```python
from build123d import *

# Parameters (mm, degrees)
EXTRUIR1_DEPTH = 2.5
REDONDEO1_R    = 10
CROQUIS2_R     = 2.5
EXTRUIR2_DEPTH = 10
REDONDEO2_R    = 5
CROQUIS4_W     = 40
CROQUIS4_H     = 5
EXTRUIR3_DEPTH = 10


with BuildPart() as part:
    # Croquis1 → Extruir1 (new, symmetric)
    with BuildSketch(Plane.XY):
        with BuildLine():
            Line((78.941483087, 11.999998301), (18.941483087, 11.999994988))
            Line((18.941483087, 11.999994988), (-17.269168309, 23.774653719))
            ThreePointArc((-17.269168309, 23.774653719), (-49.603355409, 4.435638782), (-26.058513909, -24.977582614))
            Line((-26.058513909, -24.977582614), (78.941483697, -25.000001699))
            Line((78.941483697, -25.000001699), (78.941483697, -1.699e-06))
            Line((78.941483697, -1.699e-06), (78.941483087, 11.999998301))
        make_face()
    extrude(amount=EXTRUIR1_DEPTH, both=True)

    # Redondeo1
    redondeo1_edges = [part.edges().sort_by_distance(p)[0] for p in [
        (18.941483087, 11.999994988, 0),
    ]]
    fillet(redondeo1_edges, radius=REDONDEO1_R)

    # Croquis2 → Extruir2 (cut)
    with BuildSketch(Plane.XY.offset(2.5)):
        with Locations((-25.000000078, -1.697e-06)):
            Circle(CROQUIS2_R)
    extrude(amount=-EXTRUIR2_DEPTH, mode=Mode.SUBTRACT)

    # Redondeo2
    redondeo2_edges = [part.edges().sort_by_distance(p)[0] for p in [
        (78.941483697, -25.000001699, 0),
        (78.941483087, 11.999998301, 0),
    ]]
    fillet(redondeo2_edges, radius=REDONDEO2_R)

    # Croquis4 → Extruir3 (cut)
    with BuildSketch(Plane.XY.offset(2.5)):
        with Locations((53.941483697, -17.498934009)):
            Rectangle(CROQUIS4_W, CROQUIS4_H)
    extrude(amount=-EXTRUIR3_DEPTH, mode=Mode.SUBTRACT)


solid = part.part
```
Can you work these out from the model? Positions are in its coordinate system, mm. A direction names the side the tool comes from. Round coordinates to 2 decimals unless told otherwise and drop trailing zeros. Loops run counter-clockwise (first coordinate to the right, second up) from the corner with the lowest first, then second, coordinate; pieces in that order, holes last.
Item 1: Suppose I cut it at C-C, the plane y = -21.5. Write out the boundary of the cut face in (x, z).
Item 2: Suppose I cut it at B-B, the plane x = 51. Write out the boundary of the cut face in (y, z).
Item 3: Which directions (+Z, -Z, +X, -X, +Y, -Y) give clear straight access to the entire face, cutting with the end or side of a thin tool? Please do faces 5 (the flat face through (73.941, -18, 0)), 6 (the flat face through (48, 12, 0)), 7 (the flat face through (14, -5, -2.5)).
Item 4: Please list where these lines run through material, in increasing order: L1, parallel to Y at x = -25, z = 0.75; L2, parallel to Y at x = 64.5, z = -2; L3, parallel to Y at x = -37, z = 1.45.
Item 5: Suppose I cut it at D-D, the plane y = -12.5. Write out the boundary of the cut face in (x, z), then the cut area to 3 significant figures.
Item 6: Will these pins go through, and if not, where does the flat tip stop? pin 1 Ø2.5 at (x, z) = (59, -1) entering from -Y; pin 2 Ø1.5 at (x, z) = (50, -0.5) entering from +Y; pin 3 Ø2.5 at (y, z) = (-18.5, 0) entering from -X.
Item 7: Suppose I cut it at A-A, the plane z = -0.3. Write out the boundary of the cut face in (x, y), then the cut area to 3 significant figures.
Item 8: If we mould it in two halves opening along X, with no side actions, what happens to faces 1 (the flat face through (54, -14.999, 0)), 2 (the cylindrical face through (77.44, 10.57, -0.04)), 3 (the flat face through (33.941, -18, 0)), 4 (the flat face through (14, -5, 2.5))? For each: +X half, -X half, draft (parallel to the pull), parting line (faces both ways), or undercut.
Reported:
1. outline: (-37.76, -2.5) - (78.71, -2.5) - (78.71, 2.5) - (-37.76, 2.5) - close
2. outline: (-24.99, -2.5) - (-20, -2.5) - (-20, 2.5) - (-24.99, 2.5) - close; (-15, -2.5) - (12, -2.5) - (12, 2.5) - (-15, 2.5) - close
3. face 5: +Z, -Z
3. face 6: +Z, -Z, +X, +Y
3. face 7: -Z, +X, -X, +Y, -Y
4. L1: y = -24.98 to -2.5, 2.5 to 25
4. L2: y = -25 to -20, -15 to 12
4. L3: y = -21.93 to 21.93
5. outline: (-46.65, -2.5) - (78.94, -2.5) - (78.94, 2.5) - (-46.65, 2.5) - close
5. area: 628 mm2
6. pin 1: stops at y = -25
6. pin 2: stops at y = 12
6. pin 3: stops at x = -43.1
7. outline: (-26.06, -24.98) - (73.94, -25) arc R5 ccw to (78.94, -20) - (78.94, 7) arc R5 ccw to (73.94, 12) - (20.53, 12) arc R10 cw to (17.43, 12.49) - (-17.27, 23.77) arc R25 ccw (long way) to start; hole circle Ø5 at (-25, 0); hole (33.94, -20) - (73.94, -20) - (73.94, -15) - (33.94, -15) - close
7. area: 4,910 mm2
8. face 1: undercut
8. face 2: +X half
8. face 3: undercut
8. face 4: draft
